Work out the finished part from the listing and answer in its coordinate system (mm). A direction names the side the tool comes from. Round coordinates to 2 decimals unless told otherwise and drop trailing zeros. Loops run counter-clockwise (first coordinate to the right, second up) from the corner with the lowest first, then second, coordinate; pieces in that order, holes last. Notation, with made-up numbers: (-7.5, -3.75) - (22.5, -3.75) arc R27 ccw to (22.5, 29.25) - close; hole circle Ø4 at (82.5, 1.5). An arc over 180 degrees is marked (long way). Answer as CSV lines item,"result". Start each with the question number.
```python
from build123d import *

# Parameters (mm, degrees)
SKETCH1_R            = 75
BOSS_EXTRUDE1_DEPTH  = 5
SKETCH2_R            = 75
SKETCH2_R_2          = 65
BOSS_EXTRUDE2_DEPTH  = 47
SKETCH3_R            = 2.5
CUT_EXTRUDE1_DEPTH   = 16
CUT_EXTRUDE2_REACH   = 54
SKETCH4_R            = 1.5
SKETCH6_R            = 60
CUT_EXTRUDE3_DEPTH   = 47
SKETCH7_R            = 75
SKETCH7_R_2          = 65
BOSS_EXTRUDE3_DEPTH  = 2
CUT_SWEEP1_PROFILE_R = 2.9


with BuildPart() as part:
    # Sketch1 → Boss-Extrude1 (new body)
    with BuildSketch(Plane(origin=(0, 0, 0), x_dir=(1, 0, 0), z_dir=(0, 1, 0))):
        Circle(SKETCH1_R)
    extrude(amount=BOSS_EXTRUDE1_DEPTH)

    # Sketch2 → Boss-Extrude2 (add)
    with BuildSketch(Plane(origin=(0, 5, 0), x_dir=(1, 0, 0), z_dir=(0, 1, 0))):
        Circle(SKETCH2_R)
        Circle(SKETCH2_R_2, mode=Mode.SUBTRACT)
    extrude(amount=BOSS_EXTRUDE2_DEPTH)

    # Sketch3 → Cut-Extrude1 (cut)
    with BuildSketch(Plane(origin=(0, 52, 0), x_dir=(1, 0, 0), z_dir=(0, 1, 0))):
        with Locations((0, 70)):
            Circle(SKETCH3_R)
        with Locations((60.621778265, 35)):
            Circle(SKETCH3_R)
        with Locations((60.621778265, -35)):
            Circle(SKETCH3_R)
        with Locations((0, -70)):
            Circle(SKETCH3_R)
        with Locations((-60.621778265, -35)):
            Circle(SKETCH3_R)
        with Locations((-60.621778265, 35)):
            Circle(SKETCH3_R)
    extrude(amount=-CUT_EXTRUDE1_DEPTH, mode=Mode.SUBTRACT)

    # Sketch4 → Cut-Extrude2 (cut, up to next)
    with BuildSketch(Plane.XZ, mode=Mode.PRIVATE) as cut_extrude2_sk1:
        Circle(SKETCH4_R)
    cut_extrude2_tool1 = extrude(cut_extrude2_sk1.sketch, amount=-CUT_EXTRUDE2_REACH, mode=Mode.PRIVATE) & part.part
    add(cut_extrude2_tool1.solids().sort_by_distance((0, 0, 0))[0], mode=Mode.SUBTRACT)

    # Sketch6 → Cut-Extrude3 (cut)
    with BuildSketch(Plane(origin=(0, 52, 0), x_dir=(1, 0, 0), z_dir=(0, 1, 0))):
        with BuildLine():
            ThreePointArc((-62.965535975, 30.583349709), (-70, 0), (-62.965535975, -30.583349709))
            ThreePointArc((-62.965535975, -30.583349709), (-56.291651246, -32.5), (-57.968725768, -39.238078863))
            ThreePointArc((-57.968725768, -39.238078863), (-35, -60.621778265), (-4.996810207, -69.821428571))
            ThreePointArc((-4.996810207, -69.821428571), (0, -65), (4.996810207, -69.821428571))
            ThreePointArc((4.996810207, -69.821428571), (35, -60.621778265), (57.968725768, -39.238078863))
            ThreePointArc((57.968725768, -39.238078863), (56.291651246, -32.5), (62.965535975, -30.583349709))
            ThreePointArc((62.965535975, -30.583349709), (70, 0), (62.965535975, 30.583349709))
            ThreePointArc((62.965535975, 30.583349709), (56.291651246, 32.5), (57.968725768, 39.238078863))
            ThreePointArc((57.968725768, 39.238078863), (35, 60.621778265), (4.996810207, 69.821428571))
            ThreePointArc((4.996810207, 69.821428571), (0, 65), (-4.996810207, 69.821428571))
            ThreePointArc((-4.996810207, 69.821428571), (-35, 60.621778265), (-57.968725768, 39.238078863))
            ThreePointArc((-57.968725768, 39.238078863), (-56.291651246, 32.5), (-62.965535975, 30.583349709))
        make_face()
        Circle(SKETCH6_R, mode=Mode.SUBTRACT)
    extrude(amount=-CUT_EXTRUDE3_DEPTH, mode=Mode.SUBTRACT)

    # Sketch7 → Boss-Extrude3 (add)
    with BuildSketch(Plane.XZ):
        Circle(SKETCH7_R)
        Circle(SKETCH7_R_2, mode=Mode.SUBTRACT)
    extrude(amount=BOSS_EXTRUDE3_DEPTH)

    # Cut-Sweep1: sweep along a path in Sketch8
    with BuildLine(Plane.XZ.offset(2)) as cut_sweep1_path:
        CenterArc((0, 0), 70, 0, 360)
    # Cut-Sweep1 profile (on start of the path) → Cut-Sweep1 (sweep, cut)
    with BuildSketch(Plane(origin=(70, -2, 0), x_dir=(1, 0, 0), z_dir=(0, 0, 1))):
        Circle(CUT_SWEEP1_PROFILE_R)
    sweep(path=cut_sweep1_path.line, mode=Mode.SUBTRACT)


solid = part.part
```
Item 1: Flat-ended cylindrical pins translate along their axes: pin 1 Ø5 at (y, z) = (29, -59.5) entering from -X; pin 2 Ø5 at (x, z) = (-49, 38) entering from -Y; pin 3 Ø1.5 at (x, z) = (61.5, 36) entering from +Y; pin 4 Ø1.8 at (x, z) = (0, 0) entering from +Y. Find the tip coordinate at first contact, or state that the pin passes through.
Item 2: Determine the mould class of faces 4 (the face through (-34.62, 28.83, -60.84)), 5 (the face through (-56, 52, -34)), 6 (the face through (-63.12, 44.11, -35.11)), 7 (the face through (-9.764, 25.378, 74.362)) for opening direction Z: pulls with the +Z half, pulls with the -Z half, needs draft (parallel to the pull), parting line crosses it, or undercut.
Item 3: Section A-A, the plane y = 7 is taken. Give the vertices of the cut face in (x, z).
Item 4: Which of the six approach directions +Z, -Z, +X, -X, +Y, -Y give full straight-line access (tool end or side, diameter ignored) to faces 1 (the face through (-35, -2, 55)), 2 (the face through (62, -0.99, 19.52)), 3 (the face through (62.93, 44.11, -34.04))?
Item 5: Find the intervals of material crossed by L1, parallel to Z at x = 0, y = 46; L2, parallel to X at y = 43.5, z = -35; L3, parallel to Z at x = -61, y = 49, in increasing order.
Answer:
1,pin 1,"stops at x = -48.74"
1,pin 2,"stops at y = 0"
1,pin 3,"stops at y = 36"
1,pin 4,"passes through"
2,face 4,"undercut"
2,face 5,"needs draft"
2,face 6,"undercut"
2,face 7,"parting line crosses it"
3,outline,"circle Ø150 at (0, 0); hole (-62.97, -30.58) arc R5 cw to (-57.97, -39.24) arc R70 ccw to (-5, -69.82) arc R5 cw to (5, -69.82) arc R70 ccw to (57.97, -39.24) arc R5 cw to (62.97, -30.58) arc R70 ccw to (62.97, 30.58) arc R5 cw to (57.97, 39.24) arc R70 ccw to (5, 69.82) arc R5 cw to (-5, 69.82) arc R70 ccw to (-57.97, 39.24) arc R5 cw to (-62.97, 30.58) arc R70 ccw to start"
4,face 1,"+Z, -Z, +X, -X, -Y"
4,face 2,"-Y"
4,face 3,"+Y"
5,L1,"z = -75 to -72.5, -67.5 to -65, 65 to 67.5, 72.5 to 75"
5,L2,"x = -66.33 to -63.12, -58.12 to -55.62, 55.62 to 58.12, 63.12 to 66.33"
5,L3,"z = -43.63 to -37.47, -32.53 to -30.01, 30.01 to 32.53, 37.47 to 43.63"
